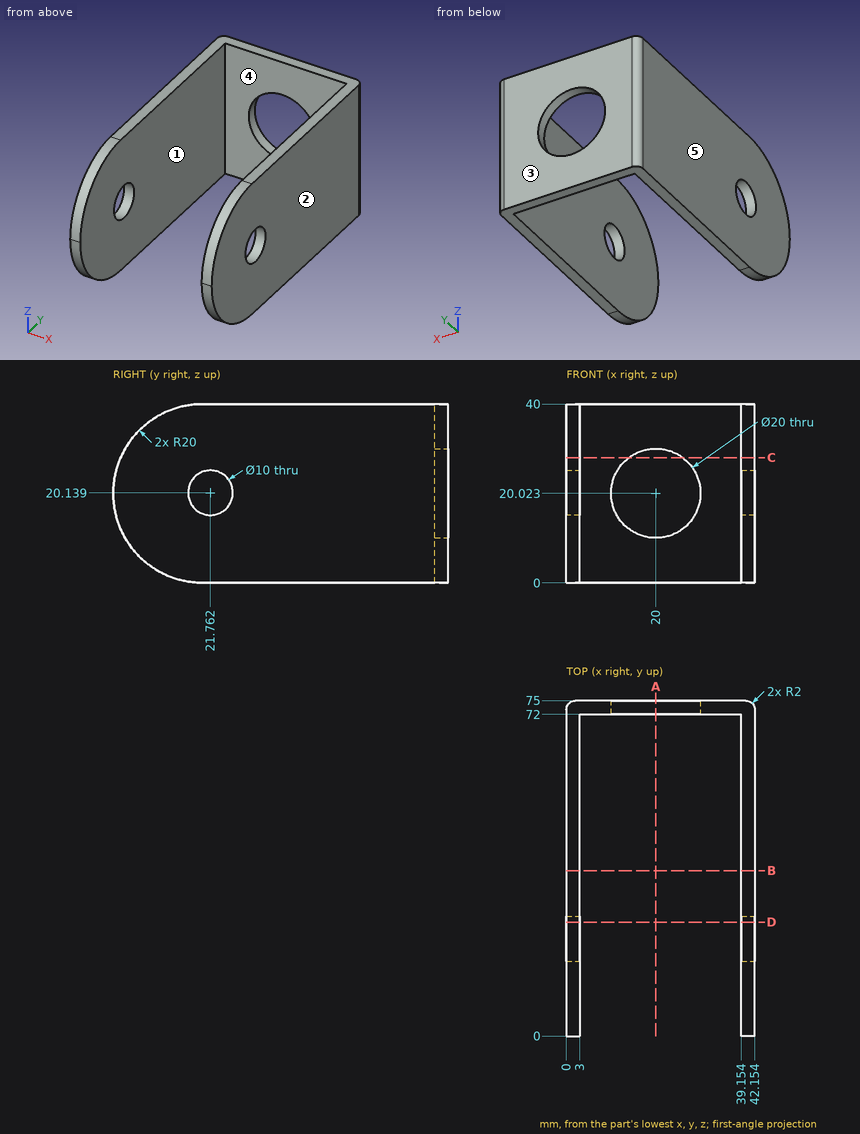
Geometry check sheet. Reference: drawing and pictorial views, mm from the part's lowest x, y, z. A direction names the side the tool comes from. Round coordinates to 2 decimals unless told otherwise and drop trailing zeros. Loops run counter-clockwise (first coordinate to the right, second up) from the corner with the lowest first, then second, coordinate; pieces in that order, holes last. Notation, with made-up numbers: (50, 29.5) - (87, 29.5) arc R22 ccw to (87, 68.5) - close; hole circle Ø7 at (67, -37.75). An arc over 180 degrees is marked (long way). Use a Markdown table: item, result. Add a question column.
1. Gauge pin test, flat end, axial feed: pin 1 (18 mm diameter, centred on x = 21, z = 27, fed in from -Y). Record the tip position at first contact, or that the pin passes through.
2. Section check A-A, the plane x = 20. Record the boundary of the cut face in (y, z), plus the area to 3 significant figures.
3. Section check D-D, the plane y = 25.5. Record the boundary of the cut face in (x, z).
4. Access from +Z, -Z, +X, -X, +Y, -Y to the whole of each face (thin tool, end or side, straight path). Record for the marked faces 4 and 5.
5. Release check for a two-part mould opening along X. For the marked faces 1, 2 and 3 record: released by +X, released by -X, zero draft, split by the parting line, or undercut.
6. Section check C-C, the plane z = 28. Record the boundary of the cut face in (x, y).
7. Section check B-B, the plane y = 37. Record the boundary of the cut face in (x, z).
8. Thickness scan on probe 1 along X at (y, z) = (29, 33.5); probe 2 along Z at (x, y) = (20, 73.85); probe 3 along Y at (x, z) = (11.5, 28). Record the ranges inside material, lowest first. Write a range as [from, to].
Checks:
| question | item | result |
|---|---|---|
| 1 | pin 1 | stops at y = 72 |
| 2 | outline | (72, 0) - (75, 0) - (75, 10.02) - (72, 10.02) - close; (72, 30.02) - (75, 30.02) - (75, 40) - (72, 40) - close |
| 2 | area | 60.0 mm^2 |
| 3 | outline | (0, 0) - (3, 0) - (3, 16.82) - (0, 16.82) - close; (0, 23.46) - (3, 23.46) - (3, 40) - (0, 40) - close; (39.15, 0) - (42.15, 0) - (42.15, 16.82) - (39.15, 16.82) - close; (39.15, 23.46) - (42.15, 23.46) - (42.15, 40) - (39.15, 40) - close |
| 4 | face 4 | +Z, -Z, -Y |
| 4 | face 5 | +Z, -Z, -X, +Y, -Y |
| 5 | face 1 | undercut |
| 5 | face 2 | released by +X |
| 5 | face 3 | zero draft |
| 6 | outline | (0, 1.67) - (3, 1.67) - (3, 72) - (13.97, 72) - (13.97, 75) - (2, 75) arc R2 ccw to (0, 73) - close; (26.03, 72) - (39.15, 72) - (39.15, 1.67) - (42.15, 1.67) - (42.15, 73) arc R2 ccw to (40.15, 75) - (26.03, 75) - close |
| 7 | outline | (0, 0) - (3, 0) - (3, 40) - (0, 40) - close; (39.15, 0) - (42.15, 0) - (42.15, 40) - (39.15, 40) - close |
| 8 | probe 1 | x = [0, 3], [39.15, 42.15] |
| 8 | probe 2 | z = [0, 10.02], [30.02, 40] |
| 8 | probe 3 | y = [72, 75] |
